Verification items for the finished model (mm, model axes). A direction names the side the tool comes from. Coordinates: 2 decimals unless noted, no trailing zeros. Order: outer loops, then holes, each group sorted by start corner. A loop starts at its lowest first (then second) coordinate and runs counter-clockwise, first axis right, second up. Notation, with made-up numbers: (3.25, 3.5) - (56.25, 3.5) arc R28 cw to (56.25, 31.5) - close; hole circle Ø1 at (41.25, 68). An arc over 180 degrees is marked (long way). Answer as CSV lines item,"result". Start each with the question number.
1. Section check A-A (y = -32). Record the cut outline in (x, z), and give its area (3 significant figures).
2. Section check B-B (z = 9). Record the cut outline in (x, y).
3. Material ranges on L1, parallel to Z at x = 16, y = -36.5; L2, parallel to Z at x = -28, y = -18; L3, parallel to X at y = -26.5, z = 25, recorded low to high. Write a range as [from, to].
4. Set-up check for faces 5 (the flat face through (25, -38, -22.475)), 6 (the cylindrical face through (59.262, -46.981, -28.736)): record each of +Z, -Z, +X, -X, +Y, -Y from which the full face is reachable in a straight line by a thin tool's end or side.
5. Go/stop test with flat-tipped pins: pin 1 (4 mm diameter, centred on x = -17, y = -7.5, fed in from +Z); pin 2 (10 mm diameter, centred on y = -41.5, z = 32.5, fed in from -X); pin 3 (5 mm diameter, centred on x = -15.5, y = -20, fed in from +Z). Record where each tip stops, or that it passes through.
6. Mould release check, pull along Z, two halves, no side actions. Record for faces 1 (the cylindrical face through (-31.889, -25.044, 26.334)), 2 (the flat face through (-64.116, -25, -9)), 3 (the flat face through (-15.8, -37.92, 23.95)), 4 (the flat face through (-2, -25, -35.175)): pulls with the +Z half, pulls with the -Z half, needs draft (parallel to the pull), parting line crosses it, or undercut.
7. Section check C-C (y = -45.5). Record the cut outline in (x, z).
8. Section check D-D (z = -1). Record the cut outline in (x, y).
from build123d import *

# Parameters (mm, degrees)
F0_R     = 12.7
F1_DEPTH = 25.4
F2_R     = 12.7
F3_DEPTH = 25.4
F4_R     = 12.7


with BuildPart() as f1:
    # F0 (on Front) → F1 (new body)
    with BuildSketch(Plane.XZ):
        with BuildLine():
            Line((62.883959, -22.474932), (-24.478167, 36.659396))
            ThreePointArc((-24.478167, 36.659396), (-50.6223, 38.061667), (-64.116041, 15.625068))
            Line((-64.116041, 15.625068), (-64.116041, -35.174932))
            Line((-64.116041, -35.174932), (62.883959, -35.174932))
            Line((62.883959, -35.174932), (62.883959, -22.474932))
        make_face()
        with Locations((-38.716041, 15.625068)):
            Circle(F0_R, mode=Mode.SUBTRACT)
    extrude(amount=F1_DEPTH)

    # F2 (on face) → F3 (join)
    with BuildSketch(Plane.XZ.offset(25.4)):
        with BuildLine():
            Line((62.883959, -35.174932), (62.883959, -22.474932))
            Line((62.883959, -22.474932), (-13.316041, -22.474932))
            Line((-13.316041, -22.474932), (-13.316041, 15.625068))
            Line((-13.316041, 15.625068), (-18.351755, 32.512504))
            Line((-18.351755, 32.512504), (-24.478167, 36.659396))
            ThreePointArc((-24.478167, 36.659396), (-50.6223, 38.061667), (-64.116041, 15.625068))
            Line((-64.116041, 15.625068), (-64.116041, -22.474932))
            Line((-64.116041, -22.474932), (-64.116041, -35.174932))
            Line((-64.116041, -35.174932), (62.883959, -35.174932))
        make_face()
        with Locations((-38.716041, 15.625068)):
            Circle(F2_R, mode=Mode.SUBTRACT)
    extrude(amount=F3_DEPTH)

    # F4
    f4_edges = [f1.edges().sort_by_distance(p)[0] for p in [
        (62.883959, -50.8, -28.824932),
    ]]
    fillet(f4_edges, radius=F4_R)


solid = f1.part
Evaluation:
1,outline,"(-64.12, -35.17) - (62.88, -35.17) - (62.88, -22.47) - (-13.32, -22.47) - (-13.32, 15.63) - (-18.35, 32.51) - (-24.48, 36.66) arc R25.4 ccw to (-64.12, 15.63) - close; hole circle Ø25.4 at (-38.72, 15.63)"
1,area,"4,050 mm²"
2,outline,"(-64.12, -50.8) - (-49.55, -50.8) - (-49.55, 0) - (-64.12, 0) - close; (-27.88, -50.8) - (-13.32, -50.8) - (-13.32, -25.4) - (16.38, -25.4) - (16.38, 0) - (-27.88, 0) - close"
3,L1,"z = [-35.17, -22.47]"
3,L2,"z = [-35.17, 8.81], [22.44, 38.65]"
3,L3,"x = [-62.32, -47.28], [-30.15, -16.11]"
4,face 5,"+Z, +X, -Y"
4,face 6,"+Z, -Z, +X, -Y"
5,pin 1,"stops at z = 32.95"
5,pin 2,"stops at x = -61.17"
5,pin 3,"stops at z = 32.27"
6,face 1,"undercut"
6,face 2,"needs draft"
6,face 3,"pulls with the +Z half"
6,face 4,"pulls with the -Z half"
7,outline,"(-64.12, -35.17) - (60.51, -35.17) - (60.51, -22.47) - (-13.32, -22.47) - (-13.32, 15.63) - (-18.35, 32.51) - (-24.48, 36.66) arc R25.4 ccw to (-64.12, 15.63) - close; hole circle Ø25.4 at (-38.72, 15.63)"
8,outline,"(-64.12, -50.8) - (-13.32, -50.8) - (-13.32, -25.4) - (31.16, -25.4) - (31.16, 0) - (-64.12, 0) - close"
